```python
from build123d import *

# Parameters (mm, degrees)
PAD_DEPTH    = 1
PAD001_DEPTH = 0.5


with BuildPart() as part:
    # Sketch → Pad (new body)
    with BuildSketch(Plane.XY):
        with BuildLine():
            Line((-3, -16), (3, -16))
            Line((3, -16), (3, 2))
            ThreePointArc((3, 2), (0.096514, 3.144536), (-3, 3.534144))
            Line((-3, -16), (-3, 3.534144))
        make_face()
    extrude(amount=PAD_DEPTH)

    # Sketch001 → Pad001 (new body)
    with BuildSketch(Plane.XY.offset(1)):
        Polygon((2.5, 1.5), (-2.5, 1.5), (-2.5, 0.5), (1.5, 0.5), (-2.5, -6.5), (-2.5, -7.5), (1.5, -7.5), (-2.5, -14.5), (-2.5, -15.5), (2.5, -15.5), (2.5, -14.5), (-1.5, -14.5), (2.5, -7.5), (2.5, -6.5), (-1.5, -6.5), (2.5, 0.5), align=None)
    extrude(amount=PAD001_DEPTH)


solid = part.part
```
CAD build for the part. Positions are in the model's coordinates, mm. A direction names the side the tool comes from. Coordinates: 2 decimals unless noted, no trailing zeros. Loops run counter-clockwise (first coordinate to the right, second up) from the corner with the lowest first, then second, coordinate; pieces in that order, holes last. Notation, with made-up numbers: (-7.75, 35) - (5.25, 35) arc R20 ccw to (5.25, 59) - close; hole circle Ø2 at (-1.5, -40). An arc over 180 degrees is marked (long way). Use CSV: the item, a comma, the result in double quotes. Start each with the question number.
Q1. 3-axis set-ups, long thin cutter, end or side, ignore diameter. For faces 5 (the flat face through (0.5, -3, 1.2)), 6 (the flat face through (-3, -6.4, 0.5)), 7 (the flat face through (-0.5, -11, 1.2)): which of +Z, -Z, +X, -X, +Y, -Y reach the whole face in a straight line?
Q2. Two-plate mould, pull along Y, no slides. Class faces 1 (the cylindrical face through (0.139, 3.134, 0.493)), 2 (the flat face through (0.5, -11, 1.2)), 3 (the flat face through (-0.5, -3, 1.2)), 4 (the flat face through (0, -6, 0)): +Y half, -Y half, draft (parallel to the pull), parting line (faces both ways), or undercut.
Q3. Cut at B-B, the plane y = -7. List the corners of the cut face in (x, z).
Q4. Drop flat-ended pins along their axis: P1, Ø0.6, axis at x = -1, z = 1.5, coming from the +Y side; P2, Ø1.8, axis at x = 0, y = -1.5, coming from the +Z side; P3, Ø0.6, axis at x = -0.5, z = 1.5, coming from the -Y side. Give the stop position or say it passes through.
Q5. Probe probe 1 along Y at (x, z) = (-1.8, 1.25) (3 decimals); probe 2 along Y at (x, z) = (-1.75, 1.45); probe 3 along Z at (x, y) = (-2.6, -5.75). List the from-to ranges inside material, lowest first. Write a range as from..to.
Q6. Cut at C-C, the plane x = 2.15. List the corners of the cut face in (y, z), then the cut area to 3 significant figures.
Q7. Cut at D-D, the plane x = 0.85. List the corners of the cut face in (y, z).
Q8. Cut at A-A, the plane z = 1.2. List the corners of the cut face in (x, y).
Here are the results:
1,face 5,"+Z, +X"
1,face 6,"+Z, -Z, -X, +Y, -Y"
1,face 7,"+Z, -X"
2,face 1,"+Y half"
2,face 2,"undercut"
2,face 3,"undercut"
2,face 4,"draft"
3,outline,"(-3, 0) - (3, 0) - (3, 1) - (2.5, 1) - (2.5, 1.5) - (-2.5, 1.5) - (-2.5, 1) - (-3, 1) - close"
4,P1,"y = 1.5"
4,P2,"z = 1.5"
4,P3,"y = -15.5"
5,probe 1,"-15.5..-13.275, -7.5..-5.275, 0.5..1.5"
5,probe 2,"-15.5..-13.19, -7.5..-5.19, 0.5..1.5"
5,probe 3,"0..1"
6,outline,"(-16, 0) - (2.42, 0) - (2.42, 1) - (1.5, 1) - (1.5, 1.5) - (-0.11, 1.5) - (-0.11, 1) - (-6.5, 1) - (-6.5, 1.5) - (-8.11, 1.5) - (-8.11, 1) - (-14.5, 1) - (-14.5, 1.5) - (-15.5, 1.5) - (-15.5, 1) - (-16, 1) - close"
6,area,"20.5 mm2"
7,outline,"(-16, 0) - (2.93, 0) - (2.93, 1) - (1.5, 1) - (1.5, 1.5) - (0.5, 1.5) - (0.5, 1) - (-0.64, 1) - (-0.64, 1.5) - (-2.39, 1.5) - (-2.39, 1) - (-6.5, 1) - (-6.5, 1.5) - (-7.5, 1.5) - (-7.5, 1) - (-8.64, 1) - (-8.64, 1.5) - (-10.39, 1.5) - (-10.39, 1) - (-14.5, 1) - (-14.5, 1.5) - (-15.5, 1.5) - (-15.5, 1) - (-16, 1) - close"
8,outline,"(-2.5, -15.5) - (2.5, -15.5) - (2.5, -14.5) - (-1.5, -14.5) - (2.5, -7.5) - (2.5, -6.5) - (-1.5, -6.5) - (2.5, 0.5) - (2.5, 1.5) - (-2.5, 1.5) - (-2.5, 0.5) - (1.5, 0.5) - (-2.5, -6.5) - (-2.5, -7.5) - (1.5, -7.5) - (-2.5, -14.5) - close"
